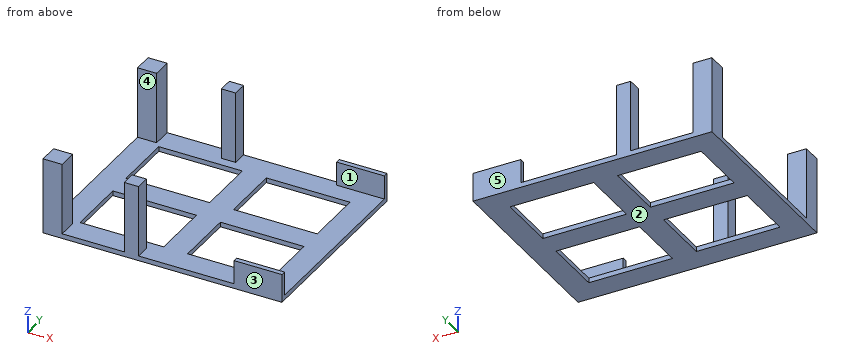
from build123d import *

# Parameters (mm, degrees)
BOX009_W     = 10
BOX009_H     = 80
BOX009_DEPTH = 2
BOX008_W     = 20
BOX008_H     = 2
BOX008_DEPTH = 12
BOX007_W     = 20
BOX007_H     = 2
BOX007_DEPTH = 12
BOX006_W     = 80
BOX006_H     = 25
BOX006_DEPTH = 10
BOX005_W     = 80
BOX005_H     = 25
BOX005_DEPTH = 10
BOX004_W     = 6
BOX004_H     = 6
BOX004_DEPTH = 32
BOX003_W     = 6
BOX003_H     = 6
BOX003_DEPTH = 32
BOX002_W     = 8
BOX002_H     = 8
BOX002_DEPTH = 32
BOX001_W     = 8
BOX001_H     = 8
BOX001_DEPTH = 32
BOX_W        = 100
BOX_H        = 80
BOX_DEPTH    = 2


with BuildPart() as cube009:
    # Box009 → Box009 (new body)
    with BuildSketch(Plane(origin=(45, 0, 0), x_dir=(1, 0, 0), z_dir=(0, 0, 1))):
        with Locations((5, 40)):
            Rectangle(BOX009_W, BOX009_H)
    extrude(amount=BOX009_DEPTH)


with BuildPart() as cube008:
    # Box008 → Box008 (new body)
    with BuildSketch(Plane(origin=(80, 78, 0), x_dir=(1, 0, 0), z_dir=(0, 0, 1))):
        with Locations((10, 1)):
            Rectangle(BOX008_W, BOX008_H)
    extrude(amount=BOX008_DEPTH)


with BuildPart() as cube007:
    # Box007 → Box007 (new body)
    with BuildSketch(Plane(origin=(80, 0, 0), x_dir=(1, 0, 0), z_dir=(0, 0, 1))):
        with Locations((10, 1)):
            Rectangle(BOX007_W, BOX007_H)
    extrude(amount=BOX007_DEPTH)


with BuildPart() as cube006:
    # Box006 → Box006 (new body)
    with BuildSketch(Plane(origin=(10, 45, 0), x_dir=(1, 0, 0), z_dir=(0, 0, 1))):
        with Locations((40, 12.5)):
            Rectangle(BOX006_W, BOX006_H)
    extrude(amount=BOX006_DEPTH)


with BuildPart() as cube005:
    # Box005 → Box005 (new body)
    with BuildSketch(Plane(origin=(10, 10, 0), x_dir=(1, 0, 0), z_dir=(0, 0, 1))):
        with Locations((40, 12.5)):
            Rectangle(BOX005_W, BOX005_H)
    extrude(amount=BOX005_DEPTH)


with BuildPart() as cube004:
    # Box004 → Box004 (new body)
    with BuildSketch(Plane(origin=(34, 74, 0), x_dir=(1, 0, 0), z_dir=(0, 0, 1))):
        with Locations((3, 3)):
            Rectangle(BOX004_W, BOX004_H)
    extrude(amount=BOX004_DEPTH)


with BuildPart() as cube003:
    # Box003 → Box003 (new body)
    with BuildSketch(Plane(origin=(34, 0, 0), x_dir=(1, 0, 0), z_dir=(0, 0, 1))):
        with Locations((3, 3)):
            Rectangle(BOX003_W, BOX003_H)
    extrude(amount=BOX003_DEPTH)


with BuildPart() as cube002:
    # Box002 → Box002 (new body)
    with BuildSketch(Plane(origin=(0, 72, 0), x_dir=(1, 0, 0), z_dir=(0, 0, 1))):
        with Locations((4, 4)):
            Rectangle(BOX002_W, BOX002_H)
    extrude(amount=BOX002_DEPTH)


with BuildPart() as cube001:
    # Box001 → Box001 (new body)
    with BuildSketch(Plane.XY):
        with Locations((4, 4)):
            Rectangle(BOX001_W, BOX001_H)
    extrude(amount=BOX001_DEPTH)


with BuildPart() as fusion006:
    # Box → Box (new body)
    with BuildSketch(Plane.XY):
        with Locations((50, 40)):
            Rectangle(BOX_W, BOX_H)
    extrude(amount=BOX_DEPTH)

    # Fusion: union Cube001
    add(cube001.part)

    # Fusion001: union Cube002
    add(cube002.part)

    # Fusion002: union Cube003
    add(cube003.part)

    # Fusion003: union Cube004
    add(cube004.part)

    # Cut: cut Cube005
    add(cube005.part, mode=Mode.SUBTRACT)

    # Cut001: cut Cube006
    add(cube006.part, mode=Mode.SUBTRACT)

    # Fusion004: union Cube007
    add(cube007.part)

    # Fusion005: union Cube008
    add(cube008.part)

    # Fusion006: union Cube009
    add(cube009.part)


solid = fusion006.part
Design review of the part built by this model. Coordinates are the model's own, in mm. Face numbers are marked on the shaded views. A direction names the side the tool comes from. Coordinates: 2 decimals unless noted, no trailing zeros. Write each loop counter-clockwise with the first axis right and the second up, starting at its lowest first coordinate (ties: lowest second). Pieces come first, ordered by that corner, then holes. Notation, with made-up numbers: (15.25, 84.5) - (51.25, 84.5) arc R23 cw to (51.25, 99.5) - close; hole circle Ø10 at (66, 49). An arc over 180 degrees is marked (long way). One line per item, written item: value.
1) For the marked faces 4 and 5, list the 3-axis set-ups (+Z, -Z, +X, -X, +Y, -Y) from which the entire face can be reached by the end or side of a thin tool; tool diameter is ignored.
Answer sheet:
face 4: +Z, +X, -X
face 5: +Z, -Z, +X, -X, +Y
2) Insertion check: pin 1 (24 mm diameter, centred on x = 38, y = 33, fed in from +Z); pin 2 (2 mm diameter, centred on y = 70.5, z = 4, fed in from +X) (1 decimal); pin 3 (1.8 mm diameter, centred on y = 76, z = 12, fed in from +X). Each pin has a flat end and moves straight along its axis. Give the tip position at first contact, or say it passes through.
Answer sheet:
pin 1: stops at z = 2
pin 2: passes through
pin 3: stops at x = 40
3) Add section D-D (x = 17.5). State the section outline as (y, z) points.
Answer sheet:
outline: (0, 0) - (10, 0) - (10, 2) - (0, 2) - close; (35, 0) - (45, 0) - (45, 2) - (35, 2) - close; (70, 0) - (80, 0) - (80, 2) - (70, 2) - close
4) Mouldability with a two-part tool opening along Y and no side actions: class the marked faces 1, 2 and 3 as +Y half, -Y half, draft (parallel to the pull), parting line (faces both ways), or undercut.
Answer sheet:
face 1: undercut
face 2: draft
face 3: -Y half
5) Add section C-C (z = 8). State the section outline as (x, y) points, plus the area to 3 significant figures.
Answer sheet:
outline: (0, 0) - (8, 0) - (8, 8) - (0, 8) - close; (0, 72) - (8, 72) - (8, 80) - (0, 80) - close; (34, 0) - (40, 0) - (40, 6) - (34, 6) - close; (34, 74) - (40, 74) - (40, 80) - (34, 80) - close; (80, 0) - (100, 0) - (100, 2) - (80, 2) - close; (80, 78) - (100, 78) - (100, 80) - (80, 80) - close
area: 280 mm2
6) Add section B-B (y = 28.5). State the section outline as (x, z) points, plus the area to 3 significant figures.
Answer sheet:
outline: (0, 0) - (10, 0) - (10, 2) - (0, 2) - close; (45, 0) - (55, 0) - (55, 2) - (45, 2) - close; (90, 0) - (100, 0) - (100, 2) - (90, 2) - close
area: 60.0 mm2
7) Add section A-A (z = 30). State the section outline as (x, y) points, plus the area to 3 significant figures.
Answer sheet:
outline: (0, 0) - (8, 0) - (8, 8) - (0, 8) - close; (0, 72) - (8, 72) - (8, 80) - (0, 80) - close; (34, 0) - (40, 0) - (40, 6) - (34, 6) - close; (34, 74) - (40, 74) - (40, 80) - (34, 80) - close
area: 200 mm2
8) To check wall thickness, follow probe 1 along X at (y, z) = (75, 8.5); probe 2 along Z at (x, y) = (9, 69). State the ranges of each line that lie inside material, in increasing order.
Answer sheet:
probe 1: x = 0 to 8, 34 to 40
probe 2: z = 0 to 2
